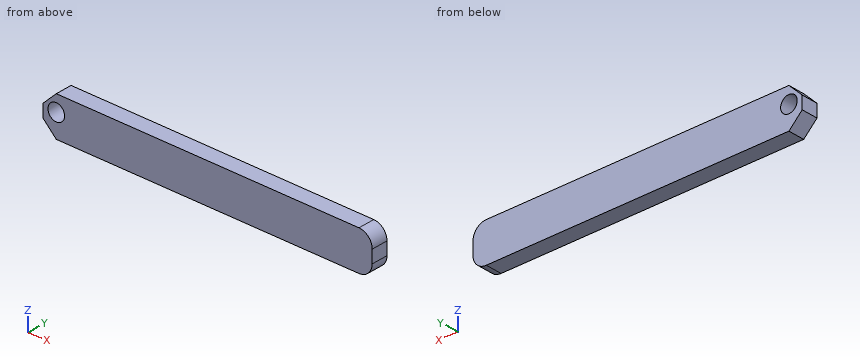
```python
from build123d import *

# Parameters (mm, degrees)
F0_W     = 125.92558
F0_H     = 15.03172
F1_DEPTH = 6.35
F2_R     = 5.08
F3_SIZE  = 5.08
F5_D     = 6.35


with BuildPart() as f1:
    # F0 (on Front) → F1 (new body)
    with BuildSketch(Plane.XZ):
        with Locations((15.213812, 20.512795)):
            Rectangle(F0_W, F0_H)
    extrude(amount=F1_DEPTH)

    # F2
    f2_edges = [f1.edges().sort_by_distance(p)[0] for p in [
        (78.176602, -3.175, 28.028655),
        (78.176602, -3.175, 12.996935),
    ]]
    fillet(f2_edges, radius=F2_R)

    # F3
    f3_edges = [f1.edges().sort_by_distance(p)[0] for p in [
        (-47.748978, -3.175, 28.028655),
        (-47.748978, -3.175, 12.996935),
    ]]
    chamfer(f3_edges, length=F3_SIZE)

    # F5 (through all)
    with Locations(Plane.XZ.offset(6.35)):
        with Locations((-42.668978, 21.895384)):
            Hole(F5_D / 2)


solid = f1.part
```
Work out the finished part from the listing and answer in its coordinate system (mm). Round coordinates to 2 decimals unless told otherwise and drop trailing zeros. Write each loop counter-clockwise with the first axis right and the second up, starting at its lowest first coordinate (ties: lowest second). Pieces come first, ordered by that corner, then holes. Notation, with made-up numbers: (-1.75, 69) - (57.25, 69) arc R14 ccw to (57.25, 95) - close; hole circle Ø11 at (-35.5, -12.75). An arc over 180 degrees is marked (long way). Return JSON: item names as keys, results as strings. Group by question number.
Q1. Find the intervals of material crossed by L1, parallel to X at y = -4.25, z = 22; L2, parallel to X at y = -1.5, z = 22.75; L3, parallel to X at y = -4.5, z = 26.75, in increasing order.
Q2. Each of these flat-tipped pins is pushed along its axis until it touches: pin 1 Ø3 at (y, z) = (-4.5, 25.5) entering from +X; pin 2 Ø5.5 at (x, z) = (-42.67, 21.9) entering from +Y. Where does it stop, or does it pass through?
Q3. The part is cut by section B-B on z = 26.75. Write down the section's boundary in (x, y), then the cut area to 3 significant figures.
Q4. The part is cut by section A-A on y = -1.5. Write down the section's boundary in (x, z) (3 decimals), then the cut area to 3 significant figures.
Solved:
{
 "1": {"L1": "-47.75 to -45.84, -39.5 to 78.18", "L2": "-47.75 to -45.73, -39.61 to 78.18", "L3": "-43.95 to 76.47"},
 "2": {"pin 1": "x = 78.07", "pin 2": "through"},
 "3": {"outline": "(-43.95, -6.35) - (76.47, -6.35) - (76.47, 0) - (-43.95, 0) - close", "area": "765 mm²"},
 "4": {"outline": "(-47.749, 18.077) - (-42.669, 12.997) - (73.097, 12.997) arc R5.08 ccw to (78.177, 18.077) - (78.177, 22.949) arc R5.08 ccw to (73.097, 28.029) - (-42.669, 28.029) - (-47.749, 22.949) - close; hole circle Ø6.35 at (-42.669, 21.895)", "area": "1,820 mm²"}
}
